```python
from build123d import *

# Parameters (mm, degrees)
SKETCH2_W               = 15
SKETCH2_H               = 37.5
BOSS_EXTRUDE1_DEPTH     = 5
SKETCH3_W               = 15
SKETCH3_H               = 5
BOSS_EXTRUDE2_DEPTH     = 20
SKETCH4_W               = 3
SKETCH4_H               = 10
BOSS_EXTRUDE3_DEPTH     = 20
CUT_EXTRUDE1_DEPTH      = 48.5
CUT_EXTRUDE1_DEPTH_BACK = 48.5
SKETCH5_R               = 1.7
FILLET1_R               = 20
SKETCH6_R               = 2.65
CUT_EXTRUDE2_DEPTH      = 10
SKETCH7_R               = 2.65
CUT_EXTRUDE3_DEPTH      = 10


with BuildPart() as part:
    # Sketch2 → Boss-Extrude1 (new body)
    with BuildSketch(Plane.XY):
        with Locations((7.5, 18.75)):
            Rectangle(SKETCH2_W, SKETCH2_H)
    extrude(amount=BOSS_EXTRUDE1_DEPTH)

    # Sketch3 → Boss-Extrude2 (add)
    with BuildSketch(Plane.XY.offset(5)):
        with Locations((7.5, 2.5)):
            Rectangle(SKETCH3_W, SKETCH3_H)
    extrude(amount=BOSS_EXTRUDE2_DEPTH)

    # Sketch4 → Boss-Extrude3 (add)
    with BuildSketch(Plane(origin=(0, 0, 0), x_dir=(-1, 0, 0), z_dir=(0, 0, -1))):
        with Locations((-13.5, 32.5)):
            Rectangle(SKETCH4_W, SKETCH4_H)
        with Locations((-1.5, 32.5)):
            Rectangle(SKETCH4_W, SKETCH4_H)
    extrude(amount=BOSS_EXTRUDE3_DEPTH)

    # Sketch5 → Cut-Extrude1 (cut, two sides: drawn at the far end of the back side and taken through both)
    with BuildSketch(Plane(origin=(15, 0, 0), x_dir=(0, 0, -1), z_dir=(1, 0, 0)).offset(-CUT_EXTRUDE1_DEPTH_BACK)):
        with Locations(Location((8.5, 32.5, 0), (0, 0, 90))):
            Circle(SKETCH5_R)
    extrude(amount=CUT_EXTRUDE1_DEPTH + CUT_EXTRUDE1_DEPTH_BACK, mode=Mode.SUBTRACT)

    # Fillet1
    fillet1_edges = [part.edges().sort_by_distance(p)[0] for p in [
        (1.5, 27.5, 0),
        (13.5, 27.5, 0),
    ]]
    fillet(fillet1_edges, radius=FILLET1_R - 0.0001)  # a hair under: the kernel refuses the full size

    # Sketch6 → Cut-Extrude2 (cut)
    with BuildSketch(Plane.XZ):
        with Locations(Location((7.5, 15, 0), (0, 0, 270))):
            Circle(SKETCH6_R)
    extrude(amount=-CUT_EXTRUDE2_DEPTH, mode=Mode.SUBTRACT)

    # Sketch7 → Cut-Extrude3 (cut)
    with BuildSketch(Plane(origin=(0, 0, 0), x_dir=(-1, 0, 0), z_dir=(0, 0, -1))):
        with Locations((-7.5, 15)):
            Circle(SKETCH7_R)
    extrude(amount=-CUT_EXTRUDE3_DEPTH, mode=Mode.SUBTRACT)


solid = part.part
```
Could you check a few things on this model? Use its own coordinates, in mm. A direction names the side the tool comes from. Round coordinates to 2 decimals unless told otherwise and drop trailing zeros. Write each loop counter-clockwise with the first axis right and the second up, starting at its lowest first coordinate (ties: lowest second). Pieces come first, ordered by that corner, then holes. Notation, with made-up numbers: M -29.5,-37.75 L 13.5,-37.75 A20 cw 13.5,-22.75 Z; hole C 48.25,11 d10. An arc over 180 degrees is marked long. Answer in a Markdown table with one row per item. Add a question column.
Q1. Will these pins go through, and if not, where does the flat tip stop? pin 1 Ø10 at (y, z) = (22, -14) entering from -X; pin 2 Ø1.5 at (x, y) = (13, 9) entering from +Z; pin 3 Ø6 at (x, z) = (7.5, 15) entering from +Y.
Q2. Imagine slicing it at B-B (y = 3.5). Please give me the cut outline in (x, z).
Q3. Imagine slicing it at A-A (x = 7.5). Please give me the cut outline in (y, z), then the cut area to 4 significant figures.
Q4. Imagine slicing it at C-C (z = 15). Please give me the cut outline in (x, y).
Q5. If we mould it in two halves opening along Y, with no side actions, what happens to faces 5 (the flat face through (2.6, 37.5, -4.5)), 6 (the flat face through (12, 29, -8)), 7 (the cylindrical face through (13.48, 34.07, -9.15))? For each: +Y half, -Y half, draft (parallel to the pull), parting line (faces both ways), or undercut.
Q6. If I drill on line 1 (X direction, y = 35, z = -4); line 2 (X direction, y = 3.45, z = 15); line 3 (Y direction, x = 4, z = 6.5), over which ranges is the centre line in solid material (lowest first)? Write a range as from..to.
Q7. On a 3-axis mill with a long thin cutter (end or side, diameter ignored), from which of +Z, -Z, +X, -X, +Y, -Y can I reach the whole of each face in a straight line? I mean faces 1 (the flat face through (14, 33, -20)), 2 (the flat face through (3, 29, -8)), 3 (the flat face through (5.7, 5, 12.6)), 4 (the flat face through (7, 19, 0)). Say none if no direction works.
Values:
| question | item | result |
|---|---|---|
| 1 | pin 1 | x = 0 |
| 1 | pin 2 | z = 5 |
| 1 | pin 3 | y = 5 |
| 2 | outline | M 0,0 L 15,0 L 15,25 L 0,25 Z; hole C 7.5,15 d5.3 |
| 3 | outline | M 0,0 L 12.35,0 L 12.35,5 L 5,5 L 5,12.35 L 0,12.35 Z; M 0,17.65 L 5,17.65 L 5,25 L 0,25 Z; M 17.65,0 L 37.5,0 L 37.5,5 L 17.65,5 Z |
| 3 | area | 234.5 mm^2 |
| 4 | outline | M 0,0 L 4.85,0 L 4.85,5 L 0,5 Z; M 10.15,0 L 15,0 L 15,5 L 10.15,5 Z |
| 5 | face 5 | +Y half |
| 5 | face 6 | draft |
| 5 | face 7 | undercut |
| 6 | line 1 | 0..3, 12..15 |
| 6 | line 2 | 0..4.85, 10.15..15 |
| 6 | line 3 | 0..5 |
| 7 | face 1 | -Z, +X, -X, +Y, -Y |
| 7 | face 2 | -Z, +Y, -Y |
| 7 | face 3 | +Z, +X, -X, +Y |
| 7 | face 4 | -Z, -Y |
